Source: CAD feature listing. Evaluate the final solid. Frame: model axes, mm. Coordinates: 2 decimals unless noted, no trailing zeros. Write each loop counter-clockwise with the first axis right and the second up, starting at its lowest first coordinate (ties: lowest second). Pieces come first, ordered by that corner, then holes. Notation, with made-up numbers: M 54.5,-35.5 L 87.5,-35.5 A15 ccw 87.5,-6.5 Z; hole C -16,56.25 d3. An arc over 180 degrees is marked long. One line per item, written item: value. Start each with the question number.
Item 1: Pin query (flat end, axial travel): P1, Ø1, axis at x = 54.5, y = 19.5, coming from the -Z side. Return the tip coordinate at first contact, or that it passes through.
Item 2: Cut plane C-C, the plane z = 119.5. Output: boundary loops of the cut face in (x, y).
Item 3: Cut plane B-B, the plane x = 50.5. Output: boundary loops of the cut face in (y, z), then the cut area to 3 significant figures.
Item 4: Mould query, pull axis X, two halves, no side actions, for faces 1 (the flat face through (0, 25, 64)), 2 (the flat face through (38, 0, 63)), 3 (the cylindrical face through (35.889, 43.685, 62.611)). Classes: released by +X, released by -X, zero draft, split by the parting line, or undercut.
Item 5: Ray query, L1, parallel to X at y = 23.5, z = 21; L2, parallel to X at y = 14, z = 25; L3, parallel to Y at x = 26, z = 93.5. Return the intervals inside material, ascending. Write a range as from..to.
Item 6: Cut plane A-A, the plane y = 33. Output: boundary loops of the cut face in (x, z), then the cut area to 3 significant figures.
Autodesk Fusion 360 part; units mm, degrees
sketch "Sketch1" plane through (0, 0, 0) normal (0, 1, 0) x (1, 0, 0)
  line L0 (0, 0) -> (76.2, 0)
  line L1 (76.2, 0) -> (76.2, -203.2)
  line L2 (76.2, -203.2) -> (0, -203.2)
  line L3 (0, -203.2) -> (0, 0)
  dimension "d1" = 76.2
  dimension "d2" = 203.2
extrude "Extrude1" add sketch "Sketch1" along normal blind 50
hole "Hole1" at (36.7688, 23.7048, 203.2) direction (0, 0, -1) diameter 40 end through all
sketch "Sketch2" plane through (0, 50, 0) normal (0, 1, 0) x (-1, 0, 0)
  line L0 (0, 203.2) -> (-76.2, 203.2)
  line L1 (-76.2, 203.2) -> (-76.2, 0)
  line L2 (-76.2, 0) -> (0, 0)
  line L3 (0, 0) -> (0, 203.2)
  line L4 (150, 0) -> (73.8, 0)
  line L5 (73.8, 0) -> (73.8, 127)
  line L6 (73.8, 127) -> (150, 127)
  line L7 (150, 127) -> (150, 0)
  dimension "d8" = 76.2
  dimension "d9" = 127
sketch "Sketch3" plane through (0, 0, 0) normal (0, 1, 0) x (1, 0, 0)
  line L0 (79.4367, 34.7313) -> (3.2367, 34.7313)
  line L1 (3.2367, 34.7313) -> (3.2367, 237.9313)
  line L2 (3.2367, 237.9313) -> (79.4367, 237.9313)
  line L3 (79.4367, 237.9313) -> (79.4367, 34.7313)
  dimension "d13" = 76.2
  dimension "d14" = 203.2
move_face "OffsetFaces1" offset -76.2 1 faces at (69.7043, 25.0665, 203.2)
From the geometry:
1. P1: passes through
2. outline: M 0,0 L 76.2,0 L 76.2,50 L 0,50 Z; hole C 36.77,23.7 d40
3. outline: M 0,0 L 9.16,0 L 9.16,127 L 0,127 Z; M 38.25,0 L 50,0 L 50,127 L 38.25,127 Z
3. area: 2,660 mm²
4. face 1: released by -X
4. face 2: zero draft
4. face 3: undercut
5. L1: x = 0..16.77, 56.77..76.2
5. L2: x = 0..19.28, 54.26..76.2
5. L3: y = 0..6.85, 40.56..50
6. outline: M 0,0 L 19.06,0 L 19.06,127 L 0,127 Z; M 54.48,0 L 76.2,0 L 76.2,127 L 54.48,127 Z
6. area: 5,180 mm²
